Job drawing, mm, ordinate dimensions from the low corner. One solid piece. A direction names the side the tool comes from. Round coordinates to 2 decimals unless told otherwise and drop trailing zeros. Write each loop counter-clockwise with the first axis right and the second up, starting at its lowest first coordinate (ties: lowest second). Pieces come first, ordered by that corner, then holes.
1) Pull direction Y, two halves, no side cores. Call the marked faces 3, 4, 5 and 6: +Y half, -Y half, draft (parallel to the pull), parting line (faces both ways), or undercut.
2) Saw through at D-D on y = 96. Write the cut outline in (x, z), and give its area (3 significant figures).
3) Drill centre lines: L1, parallel to Y at x = 7.5, z = 2.2; L2, parallel to X at y = 2.5, z = 10; L3, parallel to Y at x = 1, z = 13.5. Where is each one in solid material? Low to high.
4) Saw through at B-B on x = 4. Write the cut outline in (y, z), and give its area (3 significant figures).
5) Which spindle directions (+Z, -Z, +X, -X, +Y, -Y) get a long thin tool onto all of the face, cutting with end or side? Do the marked faces 1 and 2. Say none if no direction does.
6) Saw through at C-C on y = 80. Write the cut outline in (x, z).
7) Flat gauge pins, fed straight in: pin 1 (5.5 mm diameter, centred on x = 7.5, y = 20, fed in from +Z); pin 2 (3 mm diameter, centred on y = 38, z = 7.5, fed in from +X); pin 3 (1 mm diameter, centred on x = 9, z = 8.5, fed in from +Y). Where does each tip first touch, or does it go through?
8) Saw through at A-A on z = 14. Write the cut outline in (x, y).
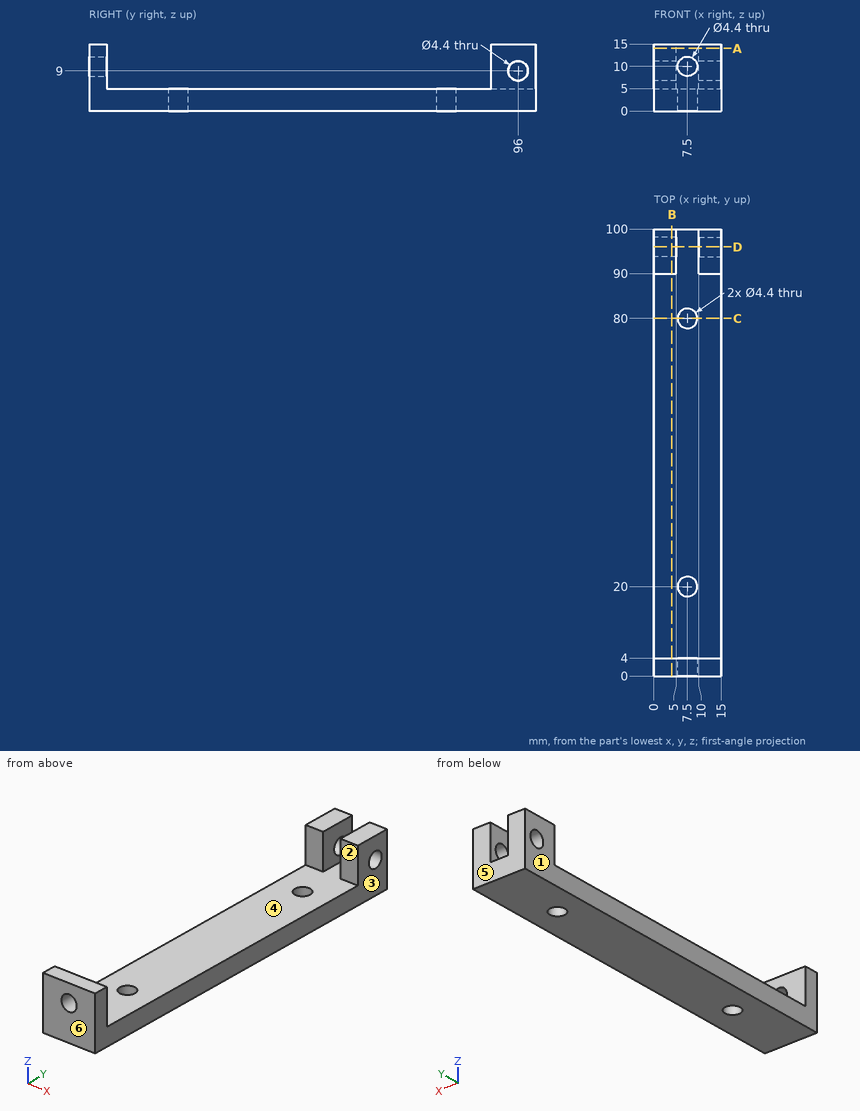
Completed:
1. face 3: draft
1. face 4: undercut
1. face 5: +Y half
1. face 6: -Y half
2. outline: (0, 0) - (15, 0) - (15, 6.8) - (10, 6.8) - (10, 5) - (5, 5) - (5, 6.8) - (0, 6.8) - close; (0, 11.2) - (5, 11.2) - (5, 15) - (0, 15) - close; (10, 11.2) - (15, 11.2) - (15, 15) - (10, 15) - close
2. area: 131 mm2
3. L1: y = 0 to 17.8, 22.2 to 77.8, 82.2 to 100
3. L2: x = 0 to 5.3, 9.7 to 15
3. L3: y = 0 to 4, 90 to 100
4. outline: (0, 0) - (100, 0) - (100, 15) - (90, 15) - (90, 5) - (4, 5) - (4, 15) - (0, 15) - close; hole circle Ø4.4 at (96, 9)
4. area: 625 mm2
5. face 1: +Z, -Z, -X, +Y, -Y
5. face 2: +Z, +X, -X
6. outline: (0, 0) - (5.3, 0) - (5.3, 5) - (0, 5) - close; (9.7, 0) - (15, 0) - (15, 5) - (9.7, 5) - close
7. pin 1: stops at z = 5
7. pin 2: passes through
7. pin 3: stops at y = 4
8. outline: (0, 0) - (15, 0) - (15, 4) - (0, 4) - close; (0, 90) - (5, 90) - (5, 100) - (0, 100) - close; (10, 90) - (15, 90) - (15, 100) - (10, 100) - close
